Print and shaded views of the part. All mm, measured from the part's lowest x, y and z. Round coordinates to 2 decimals unless told otherwise and drop trailing zeros. Order: outer loops, then holes, each group sorted by start corner. A loop starts at its lowest first (then second) coordinate and runs counter-clockwise, first axis right, second up. Notation, with made-up numbers: M -19.5,74.5 L 16.5,74.5 A31 ccw 16.5,113.5 Z; hole C -21,-23 d7. An arc over 180 degrees is marked long. Use CSV: the item, a comma, the result in double quotes.
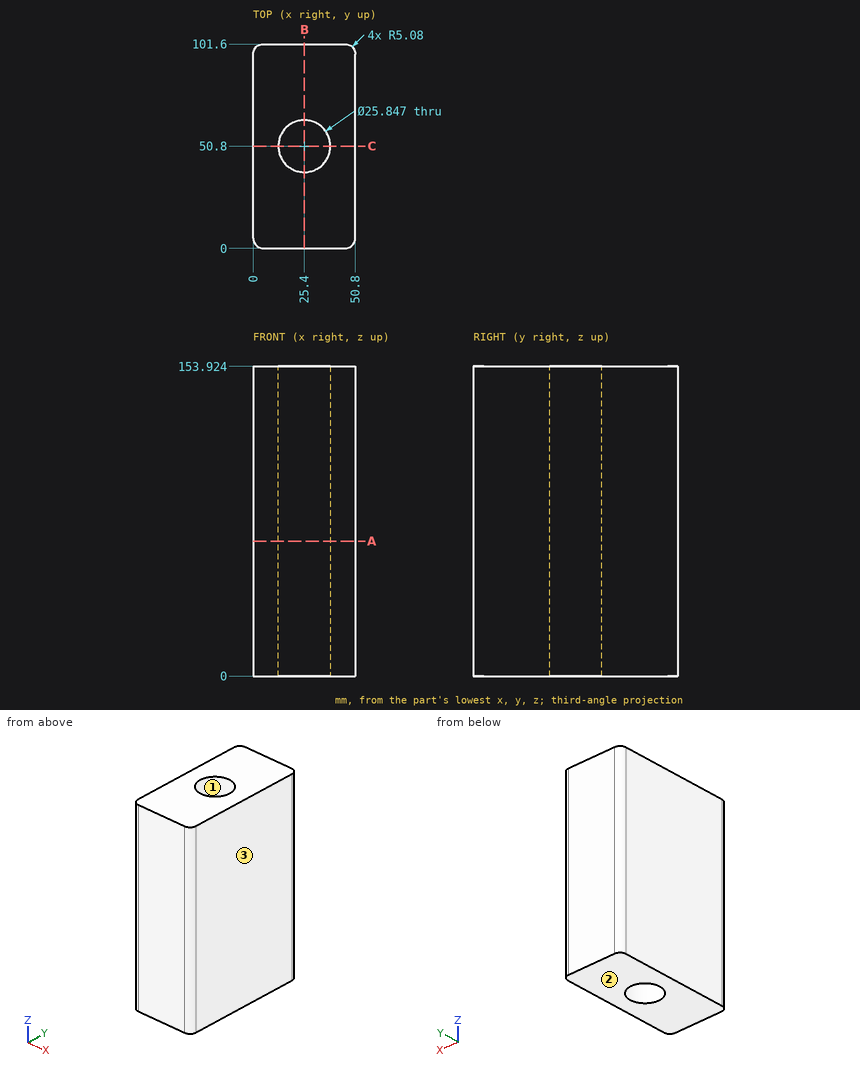
(1) Drop a flat-ended pin along its axis: pin 1 (20.5 mm diameter, centred on x = 25.4, y = 50.8, fed in from -Z). Give the stop position or say it passes through.
Answer block:
pin 1,"passes through"
(2) Two-plate mould, pull along X, no slides. Class the marked faces 1, 2 and 3: released by +X, released by -X, zero draft, split by the parting line, or undercut.
Answer block:
face 1,"undercut"
face 2,"zero draft"
face 3,"released by +X"
(3) Cut at A-A, the plane z = 67. Give the cut face in (x, y).
Answer block:
outline,"M 0,5.08 A5.08 ccw 5.08,0 L 45.72,0 A5.08 ccw 50.8,5.08 L 50.8,96.52 A5.08 ccw 45.72,101.6 L 5.08,101.6 A5.08 ccw 0,96.52 Z; hole C 25.4,50.8 d25.85"
(4) Cut at B-B, the plane x = 25.4. Give the cut face in (y, z), and give its area (3 significant figures).
Answer block:
outline,"M 0,0 L 37.88,0 L 37.88,153.92 L 0,153.92 Z; M 63.72,0 L 101.6,0 L 101.6,153.92 L 63.72,153.92 Z"
area,"11,700 mm²"
(5) Wall check: line 1 (Y direction, x = 25.4, z = 67.5); line 2 (X direction, y = 50, z = 123); line 3 (Y direction, x = 20, z = 52). Give the ranges that are in metal, low to high. Write a range as from..to.
Answer block:
line 1,"y = 0..37.88, 63.72..101.6"
line 2,"x = 0..12.5, 38.3..50.8"
line 3,"y = 0..39.06, 62.54..101.6"
(6) Cut at C-C, the plane y = 50.8. Give the cut face in (x, z).
Answer block:
outline,"M 0,0 L 12.48,0 L 12.48,153.92 L 0,153.92 Z; M 38.32,0 L 50.8,0 L 50.8,153.92 L 38.32,153.92 Z"
